Part model, mm, in its own coordinate system. A direction names the side the tool comes from. Coordinates: 2 decimals unless noted, no trailing zeros. Order: outer loops, then holes, each group sorted by start corner. A loop starts at its lowest first (then second) coordinate and runs counter-clockwise, first axis right, second up.
from build123d import *

# Parameters (mm, degrees)
SKETCH1_R               = 7.5
SKETCH1_R_2             = 4
SKETCH1_R_3             = 2.5
BOSS_EXTRUDE1_DEPTH     = 10
BOSS_EXTRUDE2_START     = 20
SKETCH1_3_R             = 7.5
SKETCH1_3_R_2           = 4
SKETCH1_3_R_3           = 2.5
BOSS_EXTRUDE2_DEPTH     = 20
CUT_EXTRUDE1_DEPTH      = 17
CUT_EXTRUDE2_DEPTH      = 23.638462845
CUT_EXTRUDE2_DEPTH_BACK = 23.638462845
SKETCH3_R               = 1.1


with BuildPart() as part:
    # Sketch1 → Boss-Extrude1 (new body)
    # profile 1 of 2: a face of its own
    with BuildSketch(Plane(origin=(0, 0, 0), x_dir=(1, 0, 0), z_dir=(0, 1, 0))):
        with Locations(Location((0, 0, 0), (0, 0, 270))):
            Circle(SKETCH1_R)
        Circle(SKETCH1_R_2, mode=Mode.SUBTRACT)
    # profile 2 of 2: a face of its own
    with BuildSketch(Plane(origin=(0, 0, 0), x_dir=(1, 0, 0), z_dir=(0, 1, 0))):
        Circle(SKETCH1_R_2)
        with Locations(Location((0, 0, 0), (0, 0, 270))):
            Circle(SKETCH1_R_3, mode=Mode.SUBTRACT)
    extrude(amount=-BOSS_EXTRUDE1_DEPTH)

    # Sketch1_3 → Boss-Extrude2 (add)
    # profile 1 of 3: a face of its own
    with BuildSketch(Plane(origin=(0, 0, 0), x_dir=(1, 0, 0), z_dir=(0, 1, 0)).offset(BOSS_EXTRUDE2_START)):
        with Locations(Location((0, 0, 0), (0, 0, 270))):
            Circle(SKETCH1_3_R)
        Circle(SKETCH1_3_R_2, mode=Mode.SUBTRACT)
    # profile 2 of 3: a face of its own
    with BuildSketch(Plane(origin=(0, 0, 0), x_dir=(1, 0, 0), z_dir=(0, 1, 0)).offset(BOSS_EXTRUDE2_START)):
        Circle(SKETCH1_3_R_2)
        with Locations(Location((0, 0, 0), (0, 0, 270))):
            Circle(SKETCH1_3_R_3, mode=Mode.SUBTRACT)
    # profile 3 of 3: a face of its own
    with BuildSketch(Plane(origin=(0, 0, 0), x_dir=(1, 0, 0), z_dir=(0, 1, 0)).offset(BOSS_EXTRUDE2_START)):
        with Locations(Location((0, 0, 0), (0, 0, 270))):
            Circle(SKETCH1_3_R_3)
    extrude(amount=-BOSS_EXTRUDE2_DEPTH)

    # Sketch2 → Cut-Extrude1 (cut)
    with BuildSketch(Plane(origin=(0, 20, 0), x_dir=(1, 0, 0), z_dir=(0, 1, 0))):
        with BuildLine():
            Line((-7.377499576, 1.35), (7.377499576, 1.35))
            ThreePointArc((7.377499576, 1.35), (7.5, 0), (7.377499576, -1.35))
            Line((7.377499576, -1.35), (-7.377499576, -1.35))
            ThreePointArc((-7.377499576, -1.35), (-7.5, 0), (-7.377499576, 1.35))
        make_face()
    extrude(amount=-CUT_EXTRUDE1_DEPTH, mode=Mode.SUBTRACT)

    # Sketch3 → Cut-Extrude2 (cut, two sides: drawn at the far end of the back side and taken through both)
    with BuildSketch(Plane.XY.offset(-CUT_EXTRUDE2_DEPTH_BACK)):
        with Locations((0, -5)):
            Circle(SKETCH3_R)
    extrude(amount=CUT_EXTRUDE2_DEPTH + CUT_EXTRUDE2_DEPTH_BACK, mode=Mode.SUBTRACT)


solid = part.part
Q1. Wall check: line 1 along X through (y, z) = (-5.25, 0); line 2 along Z through (x, y) = (-5.5, 7); line 3 along Z through (x, y) = (-0.75, 12.5). Give the ranges that are in metal, low to high.
Results list:
line 1: x = -7.5 to -2.5, 2.5 to 7.5
line 2: z = -5.1 to -1.35, 1.35 to 5.1
line 3: z = -7.46 to -1.35, 1.35 to 7.46
Q2. Which spindle directions (+Z, -Z, +X, -X, +Y, -Y) get a long thin tool onto all of the face, cutting with end or side? Do faces 1 (the face through (-2.22, -4.93, 1.15)), 2 (the face through (0, 12, 1.35)), 3 (the face through (-2, -10, -2)). Say none if no direction does.
Results list:
face 1: -Y
face 2: +X, -X, +Y
face 3: +Z, -Z, +X, -X, -Y
Q3. Cut at C-C on x = 4.5. Write the cut outline in (y, z).
Results list:
outline: (-10, -6) - (20, -6) - (20, -1.35) - (3, -1.35) - (3, 1.35) - (20, 1.35) - (20, 6) - (-10, 6) - close
Q4. Cut at D-D on y = -5. Write the cut outline in (x, z) (3 decimals).
Results list:
outline: (-1.1, -7.419) - (-1.1, -2.245) arc R2.5 cw to (-1.1, 2.245) - (-1.1, 7.419) arc R7.5 ccw to start; (1.1, -7.419) arc R7.5 ccw to (1.1, 7.419) - (1.1, 2.245) arc R2.5 cw to (1.1, -2.245) - close
Q5. Cut at A-A on x = 0. Write the cut outline in (y, z).
Results list:
outline: (-10, -7.5) - (-6.1, -7.5) - (-6.1, -2.5) - (-10, -2.5) - close; (-10, 2.5) - (-6.1, 2.5) - (-6.1, 7.5) - (-10, 7.5) - close; (-3.9, -7.5) - (20, -7.5) - (20, -1.35) - (3, -1.35) - (3, 1.35) - (20, 1.35) - (20, 7.5) - (-3.9, 7.5) - (-3.9, 2.5) - (0, 2.5) - (0, -2.5) - (-3.9, -2.5) - close
Q6. Pin check, flat tips, straight feed: pin 1 Ø2 at (y, z) = (-4.5, 4) entering from -X; pin 2 Ø1.5 at (y, z) = (12, -4.5) entering from -X; pin 3 Ø2.5 at (x, z) = (0, 0) entering from -Y. Stop position of each tip, or through.
Results list:
pin 1: stops at x = -6.87
pin 2: stops at x = -6.5
pin 3: stops at y = 0
Q7. Cut at B-B on z = 0. Write the cut outline in (x, y), and give its area (3 significant figures).
Results list:
outline: (-7.5, -10) - (-2.5, -10) - (-2.5, 0) - (2.5, 0) - (2.5, -10) - (7.5, -10) - (7.5, 3) - (-7.5, 3) - close
area: 145 mm2
Q8. Mould opens along Z. For faces 4 (the face through (-6.654, 5.21, 3.461)), 5 (the face through (0, 3, 0)), 6 (the face through (0, 20, -4)) say: pulls with the +Z half, pulls with the -Z half, needs draft (parallel to the pull), parting line crosses it, or undercut.
Results list:
face 4: parting line crosses it
face 5: undercut
face 6: needs draft
